Autodesk Inventor part; units mm, degrees
ref_plane "YZ Plane" through (0, 0, 0) normal (1, 0, 0) x (0, 1, 0)
ref_plane "XZ Plane" through (0, 0, 0) normal (0, 1, 0) x (-1, 0, 0)
ref_plane "XY Plane" through (0, 0, 0) normal (0, 0, 1) x (1, 0, 0)
sketch "Skizze1" plane through (0, 0, 0) normal (0, 0, 1) x (1, 0, 0)
  line L0 (-19.6, 0) -> (19.6, 0)
  line L1 (0, -19.6) -> (0, 19.6)
  circle A0 centre (0, 0) radius 14
  dimension "d0" = 28
extrude "Extrusion1" add sketch "Skizze1" along normal blind 20
chamfer "Fase1" distance 1 angle 45 1 edges at (-14, 0, 0)
sketch "Skizze2" plane through (0, 0, 20) normal (0, 0, 1) x (1, 0, 0)
  point P0 (0, 0)
  point P1 (0, 0)
hole "Bohrung1" at (0, 0, 20) direction (0, 0, -1) diameter 4.134 depth 11 tip angle 118
properties part number "Gummistopl groß" material "Stahl"
Verification items for the finished model (mm, model axes). A direction names the side the tool comes from. Give positions to 0.01 mm unless a question says otherwise; leave off trailing zeros. Write each loop counter-clockwise with the first axis right and the second up, starting at its lowest first coordinate (ties: lowest second). Pieces come first, ordered by that corner, then holes. Notation, with made-up numbers: M 72.25,51.5 L 92.25,51.5 A26 ccw 92.25,75.5 Z; hole C 37,38 d3. An arc over 180 degrees is marked long. Put each result on its own line as item: value. Start each with the question number.
1. Scan lines: line 1 along X through (y, z) = (0, 13); line 2 along Y through (x, z) = (9, 15). Record each from-to range of solid material in increasing order. Write a range as [from, to].
2. Section check B-B (z = 7). Record the cut outline in (x, y), and give its area (3 significant figures).
3. Go/stop test with flat-tipped pins: pin 1 Ø10 at (y, z) = (4, 17) entering from -X; pin 2 Ø8 at (x, z) = (-5.5, 7) entering from -Y; pin 3 Ø12 at (x, z) = (9, 14) entering from +Y; pin 4 Ø1.5 at (y, z) = (-3.5, 10) entering from -X. Record where each tip stops, or that it passes through.
4. Set-up check for faces 4 (the face through (1.26, 1.64, 14.42)), 5 (the face through (0, 0, 0)): record each of +Z, -Z, +X, -X, +Y, -Y from which the full face is reachable in a straight line by a thin tool's end or side.
5. Section check A-A (z = 14.5). Record the cut outline in (x, y).
6. Draft check along X on faces 1 (the face through (12.932, 5.362, 10.367)), 2 (the face through (0.108, -0.342, 7.974)), 3 (the face through (0, -3, 20)). Enter one of: +X half, -X half, draft (parallel to the pull), parting line (faces both ways), or undercut.
Answer list:
1. line 1: [-14, -2.07], [2.07, 14]
1. line 2: [-10.72, 10.72]
2. outline: C 0,0 d28
2. area: 616 mm2
3. pin 1: x = -14
3. pin 2: y = -13.92
3. pin 3: y = 13.67
3. pin 4: x = -13.73
4. face 4: +Z
4. face 5: -Z, +X, -X, +Y, -Y
5. outline: C 0,0 d28; hole C 0,0 d4.13
6. face 1: parting line
6. face 2: undercut
6. face 3: draft
